Could you check a few things on this drawing? It's one solid part, dimensions in mm from its lowest x, y, z. A direction names the side the tool comes from. Round coordinates to 2 decimals unless told otherwise and drop trailing zeros. Write each loop counter-clockwise with the first axis right and the second up, starting at its lowest first coordinate (ties: lowest second). Pieces come first, ordered by that corner, then holes. Notation, with made-up numbers: (34, -11.5) - (42, -11.5) arc R29 cw to (42, 21.5) - close; hole circle Ø1 at (52.5, 24.5). An arc over 180 degrees is marked (long way). Use one line per item in the form item = value. Start each with the question number.
1. I want a section at A-A, the plane y = 34. List the corners of the cut face in (x, z) for me, plus the area to 3 significant figures.
2. I want a section at B-B, the plane z = 130. List the corners of the cut face in (x, y) for me, plus the area to 3 significant figures.
3. I want a section at D-D, the plane y = 44. List the corners of the cut face in (x, z) for me, plus the area to 3 significant figures.
4. I want a section at C-C, the plane x = 55. List the corners of the cut face in (y, z) for me.
5. Will these pins go through, and if not, where does the flat tip stop? pin 1 (2 mm diameter, centred on y = 30.5, z = 104.5, fed in from -X); pin 2 (16.5 mm diameter, centred on y = 33.5, z = 162.5, fed in from +X); pin 3 (12 mm diameter, centred on y = 27, z = 164, fed in from -X).
6. If I drill on line 1 along Y through (x, z) = (30, 1.7); line 2 along Z through (x, y) = (47.5, 52); line 3 along Z through (x, y) = (22, 26), over which ranges is the centre line in solid material (lowest first)?
7. Which directions (+Z, -Z, +X, -X, +Y, -Y) give clear straight access to the entire face, cutting with the end or side of a thin tool? Please do the marked faces 1 and 2.
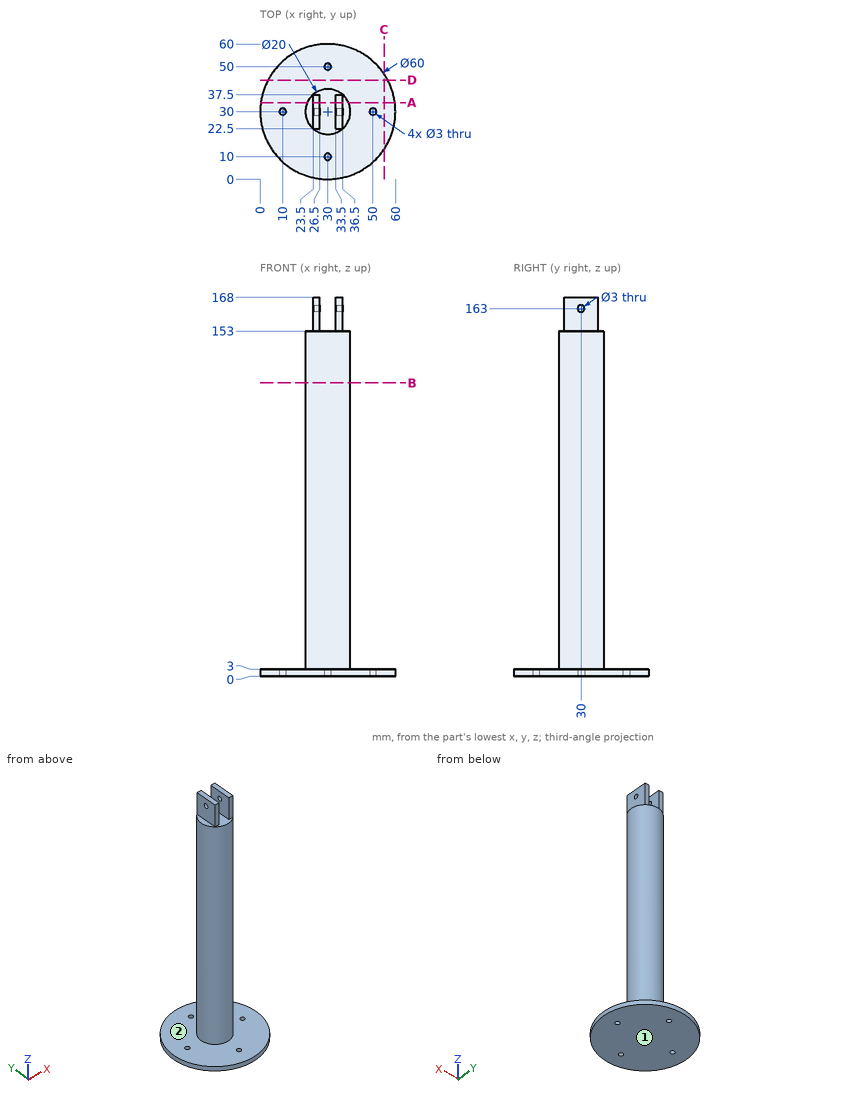
Model answer:
q1.outline = (0.27, 0) - (59.73, 0) - (59.73, 3) - (39.17, 3) - (39.17, 153) - (36.5, 153) - (36.5, 168) - (33.5, 168) - (33.5, 153) - (26.5, 153) - (26.5, 168) - (23.5, 168) - (23.5, 153) - (20.83, 153) - (20.83, 3) - (0.27, 3) - close
q1.area = 3,020 mm2
q2.outline = circle Ø20 at (30, 30)
q2.area = 314 mm2
q3.outline = (3.47, 0) - (56.53, 0) - (56.53, 3) - (3.47, 3) - close
q3.area = 159 mm2
q4.outline = (13.42, 0) - (46.58, 0) - (46.58, 3) - (13.42, 3) - close
q5.pin_1 = 20
q5.pin_2 = 36.5
q5.pin_3 = 23.5
q6.line_1 = 0 to 8.5, 11.5 to 48.5, 51.5 to 60
q6.line_2 = 0 to 3
q6.line_3 = 0 to 153
q7.face_1 = -Z, +X, -X, +Y, -Y
q7.face_2 = +Z
